```python
from build123d import *

# Parameters (mm, degrees)
SKETCH3_R           = 1.5
BOSS_EXTRUDE1_DEPTH = 3


with BuildPart() as part:
    # Sketch3 → Boss-Extrude1 (new body)
    with BuildSketch(Plane(origin=(0, 0, 0), x_dir=(1, 0, 0), z_dir=(0, 1, 0))):
        with BuildLine():
            Line((-60.745672261, 16.978901462), (-60.745672261, 18.978901462))
            ThreePointArc((-60.745672261, 18.978901462), (-60.159885823, 20.393115024), (-58.745672261, 20.978901462))
            Line((-58.745672261, 20.978901462), (-53.245672261, 20.978901462))
            ThreePointArc((-53.245672261, 20.978901462), (-51.831458698, 20.393115024), (-51.245672261, 18.978901462))
            Line((-51.245672261, 18.978901462), (-51.245672261, 16.978901462))
            ThreePointArc((-51.245672261, 16.978901462), (-49.124351917, 16.100221806), (-48.245672261, 13.978901462))
            Line((-48.245672261, 13.978901462), (-48.245672261, 10.478901462))
            Line((-48.245672261, 10.478901462), (-47.245672261, 10.478901462))
            Line((-47.245672261, 10.478901462), (-47.245672261, -1.521098538))
            Line((-47.245672261, -1.521098538), (-48.245672261, -1.521098538))
            Line((-48.245672261, -1.521098538), (-48.245672261, -5.021098538))
            ThreePointArc((-48.245672261, -5.021098538), (-49.124351917, -7.142418882), (-51.245672261, -8.021098538))
            Line((-51.245672261, -8.021098538), (-51.245672261, -10.021098538))
            ThreePointArc((-51.245672261, -10.021098538), (-51.831458698, -11.4353121), (-53.245672261, -12.021098538))
            Line((-53.245672261, -12.021098538), (-58.745672261, -12.021098538))
            ThreePointArc((-58.745672261, -12.021098538), (-60.159885823, -11.4353121), (-60.745672261, -10.021098538))
            Line((-60.745672261, -10.021098538), (-60.745672261, -8.021098538))
            Line((-60.745672261, -8.021098538), (-70.245672261, -8.021098538))
            ThreePointArc((-70.245672261, -8.021098538), (-72.366992604, -7.142418882), (-73.245672261, -5.021098538))
            Line((-73.245672261, -5.021098538), (-73.245672261, -2.521098538))
            ThreePointArc((-73.245672261, -2.521098538), (-72.659885823, -1.106884976), (-71.245672261, -0.521098538))
            Line((-71.245672261, -0.521098538), (-58.132423607, -0.521098538))
            Line((-58.132423607, -0.521098538), (-59.864474414, -3.521098538))
            Line((-59.864474414, -3.521098538), (-57.555073337, -7.521098538))
            Line((-57.555073337, -7.521098538), (-52.936271184, -7.521098538))
            Line((-52.936271184, -7.521098538), (-50.626870107, -3.521098538))
            Line((-50.626870107, -3.521098538), (-52.358920915, -0.521098538))
            Line((-52.358920915, -0.521098538), (-48.245672261, -0.521098538))
            Line((-48.245672261, -0.521098538), (-48.245672261, 9.478901462))
            Line((-48.245672261, 9.478901462), (-52.358920915, 9.478901462))
            Line((-52.358920915, 9.478901462), (-50.626870107, 12.478901462))
            Line((-50.626870107, 12.478901462), (-52.936271184, 16.478901462))
            Line((-52.936271184, 16.478901462), (-57.555073337, 16.478901462))
            Line((-57.555073337, 16.478901462), (-59.864474414, 12.478901462))
            Line((-59.864474414, 12.478901462), (-58.132423607, 9.478901462))
            Line((-58.132423607, 9.478901462), (-71.245672261, 9.478901462))
            ThreePointArc((-71.245672261, 9.478901462), (-72.659885823, 10.0646879), (-73.245672261, 11.478901462))
            Line((-73.245672261, 11.478901462), (-73.245672261, 13.978901462))
            ThreePointArc((-73.245672261, 13.978901462), (-72.366992604, 16.100221806), (-70.245672261, 16.978901462))
            Line((-70.245672261, 16.978901462), (-60.745672261, 16.978901462))
        make_face()
        with Locations((-68.245672261, -3.521098538)):
            Circle(SKETCH3_R, mode=Mode.SUBTRACT)
        with Locations((-68.245672261, 12.478901462)):
            Circle(SKETCH3_R, mode=Mode.SUBTRACT)
    extrude(amount=BOSS_EXTRUDE1_DEPTH)


solid = part.part
```
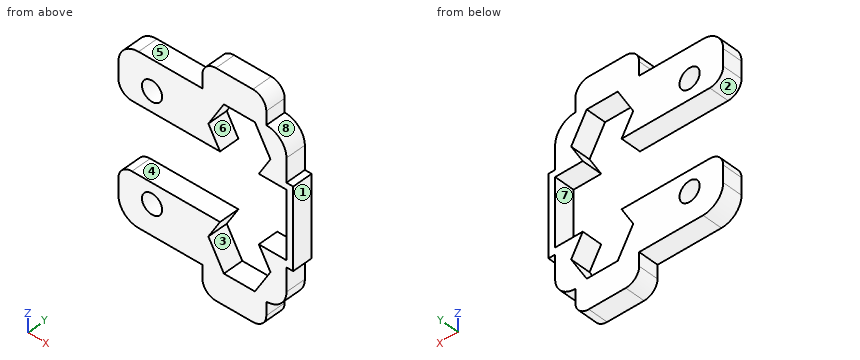
The listing builds one solid part. Answer for the finished solid, in the listing's coordinates (mm). Face numbers are marked on the shaded views. A direction names the side the tool comes from. Coordinates: 2 decimals unless noted, no trailing zeros. Write each loop counter-clockwise with the first axis right and the second up, starting at its lowest first coordinate (ties: lowest second). Pieces come first, ordered by that corner, then holes. Notation, with made-up numbers: (3, 74.5) - (46, 74.5) arc R13 ccw to (46, 84.5) - close; hole circle Ø11 at (-25.75, 63). An arc over 180 degrees is marked (long way). Return JSON: item names as keys, results as strings. Group by question number.
1. Determine the mould class of the marked faces 1, 2, 3 and 4 for opening direction X: released by +X, released by -X, zero draft, split by the parting line, or undercut.
2. A cutting plane is placed at D-D, the plane z = 9.5. Determine the outline of the cut face in (x, y), plus the area to 3 significant figures.
3. Which of the six approach directions +Z, -Z, +X, -X, +Y, -Y give full straight-line access (tool end or side, diameter ignored) to the marked faces 5, 6, 7 and 8?
4. A cutting plane is placed at B-B, the plane y = 0.35. Give the number of separate pieces and of enclosed holes in the cut face, plus the area to 3 significant figures.
5. A cutting plane is placed at A-A, the plane x = -66.25. Determine the outline of the cut face in (y, z).
6. A cutting plane is placed at C-C, the plane x = -57. Determine the outline of the cut face in (y, z), plus the area to 3 significant figures.
7. Straight lines are drawn through the part: L1, parallel to Z at x = -63.25, y = 2.6; L2, parallel to Z at x = -69.25, y = 0.6; L3, parallel to Z at x = -54.75, y = 2.7. For each, find the intervals that lie inside material, in ascending order.
8. Given pin 1 (1.6 mm diameter, centred on y = 1.5, z = -18.5, fed in from -X); pin 2 (1 mm diameter, centred on x = -66.5, y = 0.5, fed in from -Z), each flat-ended and moving along its own axis, determine where each tip first touches the part or whether it passes through.
Ans:
{
 "1": {"face 1": "released by +X", "face 2": "released by -X", "face 3": "undercut", "face 4": "zero draft"},
 "2": {"outline": "(-60.75, 0) - (-51.25, 0) - (-51.25, 3) - (-60.75, 3) - close", "area": "28.5 mm²"},
 "3": {"face 5": "+Z, -X, +Y, -Y", "face 6": "+Y, -Y", "face 7": "-X, +Y, -Y", "face 8": "+Z, +X, +Y, -Y"},
 "4": {"separate pieces": "1", "enclosed holes": "2", "area": "336 mm²"},
 "5": {"outline": "(0, -16.98) - (3, -16.98) - (3, -9.48) - (0, -9.48) - close; (0, 0.52) - (3, 0.52) - (3, 8.02) - (0, 8.02) - close"},
 "6": {"outline": "(0, -20.98) - (3, -20.98) - (3, -16.48) - (0, -16.48) - close; (0, 7.52) - (3, 7.52) - (3, 12.02) - (0, 12.02) - close", "area": "27.0 mm²"},
 "7": {"L1": "-16.98 to -9.48, 0.52 to 8.02", "L2": "-16.98 to -13.59, -11.36 to -9.48, 0.52 to 2.41, 4.64 to 8.02", "L3": "-20.98 to -16.48, 7.52 to 12.02"},
 "8": {"pin 1": "x = -60.75", "pin 2": "z = -16.98"}
}
